from build123d import *

# Parameters (mm, degrees)
SKETCH_1_W           = 23
SKETCH_1_H           = 43
EXTRUDE_1_DEPTH      = 54
SKETCH_2_OUTSIDE_W   = 39.552
SKETCH_2_OUTSIDE_H   = 59.552
SKETCH_2_OUTSIDE_W_2 = 23
SKETCH_2_OUTSIDE_H_2 = 43
SKETCH_2_OUTSIDE_W_3 = 19
SKETCH_2_OUTSIDE_H_3 = 39
CUT_EXTRUDE_1_DEPTH  = 44
SKETCH_3_W           = 27
SKETCH_3_H           = 45
SKETCH_3_W_2         = 21
SKETCH_3_H_2         = 40
EXTRUDE_2_DEPTH      = 43
SKETCH_4_R           = 3.25
CUT_EXTRUDE_2_DEPTH  = 74.416619372
SKETCH_5_W           = 8
SKETCH_5_H           = 3
CUT_EXTRUDE_3_DEPTH  = 30
SKETCH_6_R           = 2
EXTRUDE_3_DEPTH      = 2
EXTRUDE_4_DEPTH      = 10
EXTRUDE_4_DEPTH_BACK = 6
FILLET_1_R           = 2
EXTRUDE_5_DEPTH      = 30


with BuildPart() as part:
    # 草图1 → 凸台-拉伸1 (new body)
    with BuildSketch(Plane(origin=(0, 0, 0), x_dir=(1, 0, 0), z_dir=(0, 1, 0))):
        with Locations((11.5, 21.5)):
            Rectangle(SKETCH_1_W, SKETCH_1_H)
    extrude(amount=EXTRUDE_1_DEPTH)

    # 草图2 outside → 切除-拉伸1 (cut)
    # profile 1 of 2: a face of its own
    with BuildSketch(Plane.XZ):
        with Locations((11.5, -21.5)):
            Rectangle(SKETCH_2_OUTSIDE_W, SKETCH_2_OUTSIDE_H)
        with Locations((11.5, -21.5)):
            Rectangle(SKETCH_2_OUTSIDE_W_2, SKETCH_2_OUTSIDE_H_2, mode=Mode.SUBTRACT)
    # profile 2 of 2: a face of its own
    with BuildSketch(Plane.XZ):
        with Locations((11.5, -21.5)):
            Rectangle(SKETCH_2_OUTSIDE_W_3, SKETCH_2_OUTSIDE_H_3)
    extrude(amount=-CUT_EXTRUDE_1_DEPTH, mode=Mode.SUBTRACT)

    # 草图3 → 凸台-拉伸2 (add)
    with BuildSketch(Plane.XY):
        with Locations((11.5, -22.5)):
            Rectangle(SKETCH_3_W, SKETCH_3_H)
        with Locations((11.5, -22)):
            Rectangle(SKETCH_3_W_2, SKETCH_3_H_2, mode=Mode.SUBTRACT)
    extrude(amount=-EXTRUDE_2_DEPTH)

    # 草图4 → 切除-拉伸2 (cut, through all)
    with BuildSketch(Plane.ZY):
        with Locations((-31.5, 12)):
            Circle(SKETCH_4_R)
        with Locations((-11.5, 12)):
            Circle(SKETCH_4_R)
    extrude(amount=-CUT_EXTRUDE_2_DEPTH, mode=Mode.SUBTRACT)

    # 草图5 → 切除-拉伸3 (cut)
    with BuildSketch(Plane(origin=(0, 0, -43), x_dir=(-1, 0, 0), z_dir=(0, 0, -1))):
        with Locations((-11.5, -43.5)):
            Rectangle(SKETCH_5_W, SKETCH_5_H)
    extrude(amount=-CUT_EXTRUDE_3_DEPTH, mode=Mode.SUBTRACT)

    # 草图6 → 凸台-拉伸3 (add)
    with BuildSketch(Plane(origin=(0, 0, -43), x_dir=(-1, 0, 0), z_dir=(0, 0, -1))):
        Polygon((-25, -45), (-15.5, -45), (-15.5, -48), (-7.5, -48), (-7.5, -45), (2, -45), (2, -55), (-7.5, -55), (-15.5, -55), (-25, -55), align=None)
        with Locations((-16.5, -50)):
            Circle(SKETCH_6_R, mode=Mode.SUBTRACT)
        with Locations((-6.5, -50)):
            Circle(SKETCH_6_R, mode=Mode.SUBTRACT)
    extrude(amount=-EXTRUDE_3_DEPTH)

    # 草图8 → 凸台-拉伸4 (add, two sides: drawn at the far end of the back side and taken through both)
    with BuildSketch(Plane.XZ.offset(45).offset(-EXTRUDE_4_DEPTH_BACK)):
        Polygon((-8.6, -63.2), (-25.3, -63.2), (-25.3, -37), (-8.6, -37), (-2, -37), (-2, -43), (-8.6, -43), align=None)
        Polygon((-17.1, -59), (-23.3, -59), (-23.3, -59.7), (-21.2, -59.7), (-21.2, -60.5), (-23.3, -60.5), (-23.3, -62.2), (-19.6, -62.2), (-19.6, -61.1), (-18.8, -61.1), (-18.8, -62.2), (-10.6, -62.2), (-10.6, -59), (-16.3, -59), (-16.3, -60.1), (-17.1, -60.1), align=None, mode=Mode.SUBTRACT)
    extrude(amount=EXTRUDE_4_DEPTH + EXTRUDE_4_DEPTH_BACK)

    # 圆角1
    fillet_1_edges = [part.edges().sort_by_distance(p)[0] for p in [
        (15.5, -48, -42),
        (7.5, -48, -42),
    ]]
    fillet(fillet_1_edges, radius=FILLET_1_R)

    # 草图9 → 凸台-拉伸5 (add)
    with BuildSketch(Plane(origin=(0, -39, 0), x_dir=(1, 0, 0), z_dir=(0, 1, 0))):
        Polygon((-10.6, 57), (-10.6, 59), (-16.3, 59), (-16.3, 60.1), (-17.1, 60.1), (-17.1, 59), (-23.3, 59), (-23.3, 59.7), (-21.2, 59.7), (-21.2, 60.5), (-23.3, 60.5), (-23.3, 62.2), (-19.6, 62.2), (-19.6, 61.1), (-18.8, 61.1), (-18.8, 62.2), (-10.6, 62.2), (-10.6, 63.2), (-25.3, 63.2), (-25.3, 57), align=None)
    extrude(amount=EXTRUDE_5_DEPTH)


solid = part.part
Part model, mm, in its own coordinate system. A direction names the side the tool comes from. Coordinates: 2 decimals unless noted, no trailing zeros. Write each loop counter-clockwise with the first axis right and the second up, starting at its lowest first coordinate (ties: lowest second). Pieces come first, ordered by that corner, then holes. Notation, with made-up numbers: M -4.75,34 L 37.25,34 A36 ccw 37.25,73 Z; hole C -21.75,-17 d4. An arc over 180 degrees is marked long. Return JSON: item names as keys, results as strings.
1. Saw through at C-C, the plane y = 20. Write the cut outline in (x, z).
Determined:
{"outline": "M 0,-43 L 23,-43 L 23,0 L 0,0 Z; hole M 2,-41 L 21,-41 L 21,-2 L 2,-2 Z"}
2. Probe L1, parallel to Y at x = 6.5, z = -42.2; L2, parallel to Y at x = 21.5, z = -31.5; L3, parallel to X at y = 33, z = -15. List the from-to ranges inside material, lowest first.
Determined:
{"L1": "-55 to -52, -48 to -42, -2 to 54", "L2": "-45 to -42, -2 to 8.75, 15.25 to 54", "L3": "0 to 2, 21 to 23"}
3. Pull direction X, two halves, no side cores. Call faces 1 (the face through (-2, -50, -39)), 2 (the face through (0.986, 12.143, -14.747)), 3 (the face through (6.934, -51.952, -42.014)): pulls with the +X half, pulls with the -X half, needs draft (parallel to the pull), parting line crosses it, or undercut.
Determined:
{"face 1": "pulls with the +X half", "face 2": "needs draft", "face 3": "undercut"}
4. 3-axis set-ups, long thin cutter, end or side, ignore diameter. For faces 4 (the face through (0, 27, -21)), 5 (the face through (23, 27, -21)), 6 (the face through (11, -50, -41)), 7 (the face through (22, -22, -21)), 8 (the face through (-13, -32, -59)): which of +Z, -Z, +X, -X, +Y, -Y reach the whole face in a straight line?
Determined:
{"face 4": "+Z, -Z, -X, +Y", "face 5": "+Z, -Z, +X, +Y", "face 6": "+Z, +X, -Y", "face 7": "+Z, -Z", "face 8": "+Y, -Y"}
5. Saw through at D-D, the plane y = -31. Write the cut outline in (x, z).
Determined:
{"outline": "M -25.3,-63.2 L -10.6,-63.2 L -10.6,-62.2 L -18.8,-62.2 L -18.8,-61.1 L -19.6,-61.1 L -19.6,-62.2 L -23.3,-62.2 L -23.3,-60.5 L -21.2,-60.5 L -21.2,-59.7 L -23.3,-59.7 L -23.3,-59 L -17.1,-59 L -17.1,-60.1 L -16.3,-60.1 L -16.3,-59 L -10.6,-59 L -10.6,-57 L -25.3,-57 Z; M -2,-43 L 1,-43 L 1,0 L -2,0 Z; M 22,-43 L 25,-43 L 25,0 L 22,0 Z"}
6. Saw through at A-A, the plane y = -50. Count the separate pieces of the cut face and the enclosed holes in it, then the cut area to 3 significant figures.
Determined:
{"separate pieces": "3", "enclosed holes": "1", "area": "478 mm²"}
7. Flat gauge pins, fed straight in: pin 1 Ø0.6 at (y, z) = (-30.5, -59.5) entering from +X; pin 2 Ø9.5 at (x, y) = (14, 20) entering from -Z; pin 3 Ø12 at (y, z) = (-34, -21) entering from -X; pin 4 Ø4 at (y, z) = (12, -31.5) entering from +X. Where does each tip first touch, or does it go through?
Determined:
{"pin 1": "x = -16.3", "pin 2": "z = -43", "pin 3": "x = -2", "pin 4": "through"}
8. Saw through at B-B, the plane z = -26.5. Write the cut outline in (x, y), then the cut area to 3 significant figures.
Determined:
{"outline": "M -2,-45 L 7.5,-45 L 7.5,-42 L 1,-42 L 1,-2 L 22,-2 L 22,-42 L 15.5,-42 L 15.5,-45 L 25,-45 L 25,0 L 23,0 L 23,54 L 0,54 L 0,0 L -2,0 Z; hole M 2,0 L 21,0 L 21,44 L 2,44 Z", "area": "757 mm²"}
